For this review, take the finished solid that the model builds, in its own axes (mm). Round coordinates to 2 decimals unless told otherwise and drop trailing zeros. Write each loop counter-clockwise with the first axis right and the second up, starting at its lowest first coordinate (ties: lowest second). Pieces come first, ordered by that corner, then holes.
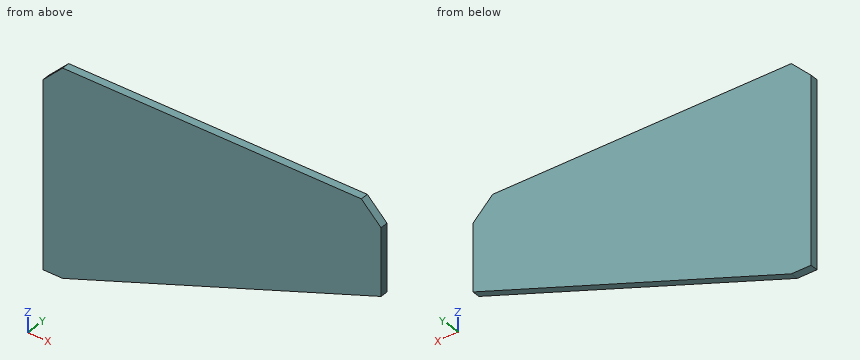
from build123d import *

# Parameters (mm, degrees)
EXTRUDE_1_DEPTH = 2
CHAMFER_2_SIZE  = 5


with BuildPart() as part:
    # Эскиз1 → Бобышка-Вытянуть1 (new body)
    with BuildSketch(Plane(origin=(0, 0, 0), x_dir=(1, 0, 0), z_dir=(0, 1, 0))):
        Polygon((5, 52), (86, 22), (86, 0), (0, 0), (0, 52), align=None)
    extrude(amount=EXTRUDE_1_DEPTH)

    # Фаска2
    chamfer_2_edges = [part.edges().sort_by_distance(p)[0] for p in [
        (0, 1, 0),
        (86, 1, 0),
    ]]
    chamfer(chamfer_2_edges, length=CHAMFER_2_SIZE)


solid = part.part
(1) For line 1 along Z through (x, y) = (43.5, 0.85); line 2 along Z through (x, y) = (76, 1.9), list the stretches that pass through material, from the lowest coordinate up.
Geometry check:
line 1: z = -37.74 to 0
line 2: z = -25.7 to 0
(2) We need section A-A, the plane y = 0.3. Give the boundary of the cut face in (x, z).
Geometry check:
outline: (0, -52) - (5, -52) - (86, -22) - (86, -5) - (81, 0) - (5, 0) - (0, -5) - close
(3) We need section C-C, the plane x = 59. Give the boundary of the cut face in (y, z).
Geometry check:
outline: (0, -32) - (2, -32) - (2, 0) - (0, 0) - close
(4) We need section B-B, the plane z = -26. Give the boundary of the cut face in (x, y), and give its area (3 significant figures).
Geometry check:
outline: (0, 0) - (75.2, 0) - (75.2, 2) - (0, 2) - close
area: 150 mm2
